Read the model definition and answer for the solid it produces. Units are mm, in the model's axes. A direction names the side the tool comes from. Give positions to 0.01 mm unless a question says otherwise; leave off trailing zeros. Write each loop counter-clockwise with the first axis right and the second up, starting at its lowest first coordinate (ties: lowest second). Pieces come first, ordered by that corner, then holes. Notation, with made-up numbers: (14, 9) -> (18, 9) arc R20 ccw to (18, 43) -> close; hole circle Ø2 at (45, 89). An arc over 180 degrees is marked (long way). Use a Markdown table: item, result.
from build123d import *

# Parameters (mm, degrees)
BOSS_EXTRUDE1_DEPTH = 76.2
SKETCH2_R           = 6.35
CUT_EXTRUDE1_DEPTH  = 28.575
SKETCH4_R           = 38.1
CUT_EXTRUDE3_DEPTH  = 83.55
SKETCH5_R           = 4.7625
CUT_EXTRUDE4_DEPTH  = 77.2000001
SKETCH6_R           = 4.7625
CUT_EXTRUDE5_DEPTH  = 28.575


with BuildPart() as part:
    # Sketch1 → Boss-Extrude1 (new body)
    with BuildSketch(Plane(origin=(0, 0, 0), x_dir=(1, 0, 0), z_dir=(0, 1, 0))):
        with BuildLine():
            Line((0, 82.55), (0, 44.45))
            ThreePointArc((0, 44.45), (44.45, 0), (0, -44.45))
            Line((0, -44.45), (0, -82.55))
            ThreePointArc((0, -82.55), (82.55, 0), (0, 82.55))
        make_face()
    extrude(amount=BOSS_EXTRUDE1_DEPTH)

    # Sketch2 → Cut-Extrude1 (cut)
    with BuildSketch(Plane.ZY):
        with Locations((-63.5, 57.15)):
            Circle(SKETCH2_R)
        with Locations((-63.5, 19.05)):
            Circle(SKETCH2_R)
        with Locations((63.5, 19.05)):
            Circle(SKETCH2_R)
        with Locations((63.5, 57.15)):
            Circle(SKETCH2_R)
    extrude(amount=-CUT_EXTRUDE1_DEPTH, mode=Mode.SUBTRACT)

    # Sketch4 → Cut-Extrude3 (cut, through all)
    with BuildSketch(Plane.ZY):
        with Locations((0, 78.74)):
            Circle(SKETCH4_R)
    extrude(amount=-CUT_EXTRUDE3_DEPTH, mode=Mode.SUBTRACT)

    # Sketch5 → Cut-Extrude4 (cut, through all)
    with BuildSketch(Plane(origin=(0, 0, 0), x_dir=(-1, 0, 0), z_dir=(0, -1, 0))):
        with Locations((-63.5, 0)):
            Circle(SKETCH5_R)
    extrude(amount=-CUT_EXTRUDE4_DEPTH, mode=Mode.SUBTRACT)

    # Sketch6 → Cut-Extrude5 (cut)
    with BuildSketch(Plane(origin=(0, 76.2, 0), x_dir=(1, 0, 0), z_dir=(0, 1, 0))):
        with Locations((38.1, -53.975)):
            Circle(SKETCH6_R)
        with Locations((38.1, 53.975)):
            Circle(SKETCH6_R)
    extrude(amount=-CUT_EXTRUDE5_DEPTH, mode=Mode.SUBTRACT)


solid = part.part
Item 1: Straight lines are drawn through the part: line 1 along Y through (x, z) = (21, 63); line 2 along Z through (x, y) = (38, 65); line 3 along Z through (x, y) = (23, 65). For each, find the intervals that lie inside material, in ascending order. Write a range as [from, to].
Return value:
| item | result |
|---|---|
| line 1 | [0, 12.72], [25.38, 50.82], [63.48, 76.2] |
| line 2 | [-73.28, -58.74], [-49.21, -35.54], [35.54, 49.21], [58.74, 73.28] |
| line 3 | [-79.28, -38.04], [38.04, 79.28] |
Item 2: A cutting plane is placed at A-A (z = 0). Give the vertices of the cut face in (x, y).
Return value:
| item | result |
|---|---|
| outline | (44.45, 0) -> (58.74, 0) -> (58.74, 40.64) -> (44.45, 40.64) -> close; (68.26, 0) -> (82.55, 0) -> (82.55, 40.64) -> (68.26, 40.64) -> close |
Item 3: For a pull along Y with two mould halves and no side action, classify faces 4 (the face through (50, 0, -1)), 5 (the face through (68.258, 20.183, -0.209)), 6 (the face through (28.575, 19, -64)), 7 (the face through (38, 47.625, -54)) as +Y half, -Y half, draft (parallel to the pull), parting line (faces both ways), or undercut.
Return value:
| item | result |
|---|---|
| face 4 | -Y half |
| face 5 | draft |
| face 6 | undercut |
| face 7 | +Y half |
Item 4: A cutting plane is placed at B-B (y = 70). Count the separate pieces of the cut face and the enclosed holes in it, then the cut area to 3 significant figures.
Return value:
| item | result |
|---|---|
| separate pieces | 2 |
| enclosed holes | 2 |
| area | 4,410 mm^2 |
Item 5: A tool of negligible diameter and unlimited length cuts with its end or side. For faces 1 (the face through (38, 47.625, 54)), 2 (the face through (28, 76.2, -56)), 3 (the face through (28.575, 57, 63)), from which of +Z, -Z, +X, -X, +Y, -Y can it reach the whole face along a straight path? Write none if from no direction.
Return value:
| item | result |
|---|---|
| face 1 | +Y |
| face 2 | +Z, -Z, +X, -X, +Y |
| face 3 | -X |
Item 6: A cutting plane is placed at C-C (x = 26.5). Give the vertices of the cut face in (y, z).
Return value:
| item | result |
|---|---|
| outline | (0, -78.18) -> (76.2, -78.18) -> (76.2, -38.02) arc R38.1 cw to (65.4, -35.69) -> (0, -35.69) -> close; (0, 35.69) -> (65.4, 35.69) arc R38.1 cw to (76.2, 38.02) -> (76.2, 78.18) -> (0, 78.18) -> close; hole circle Ø12.7 at (19.05, -63.5); hole circle Ø12.7 at (19.05, 63.5); hole circle Ø12.7 at (57.15, -63.5); hole circle Ø12.7 at (57.15, 63.5) |
Item 7: Each of these flat-tipped pins is pushed along its axis until it touches: P1, Ø10, axis at y = 43, z = -14, coming from the +X side; P2, Ø6.5, axis at y = 19, z = -61, coming from the -X side (3 decimals); P3, Ø8.5, axis at x = 38.1, z = 53.975, coming from the +Y side (3 decimals); P4, Ø8.5, axis at x = 63.5, z = 0, coming from the +Y side. Where does it stop, or does it pass through?
Return value:
| item | result |
|---|---|
| P1 | x = 82.04 |
| P2 | x = 28.575 |
| P3 | y = 47.625 |
| P4 | through |
